Geometry: see drawing. Coordinates: mm, zero at the bounding-box minimum. Round coordinates to 2 decimals unless told otherwise and drop trailing zeros. Loops run counter-clockwise (first coordinate to the right, second up) from the corner with the lowest first, then second, coordinate; pieces in that order, holes last.
(1) Line query: line 1 (X direction, y = 3.75, z = 179) (1 decimal); line 2 (Z direction, x = 157, y = 5) (1 decimal); line 3 (X direction, y = 2.5, z = 171.5) (1 decimal). Output: solid intervals per line, ascending.
(2) First-contact query: pin 1 Ø4 at (x, z) = (17.46, 119.06) entering from +Y; pin 2 Ø6 at (x, z) = (41, 180.5) entering from -Y; pin 3 Ø3 at (y, z) = (2, 55) entering from -X; pin 4 Ø3 at (x, y) = (37, 3) entering from -Z (1 decimal). Flat tips, straight axial feed; report the tip coordinate or a pass-through.
(3) Cut plane C-C, the plane y = 1.25. Output: boundary loops of the cut face in (x, z) (1 decimal), and give its area (3 significant figures).
(4) Cut plane D-D, the plane z = 206. Output: boundary loops of the cut face in (x, y).
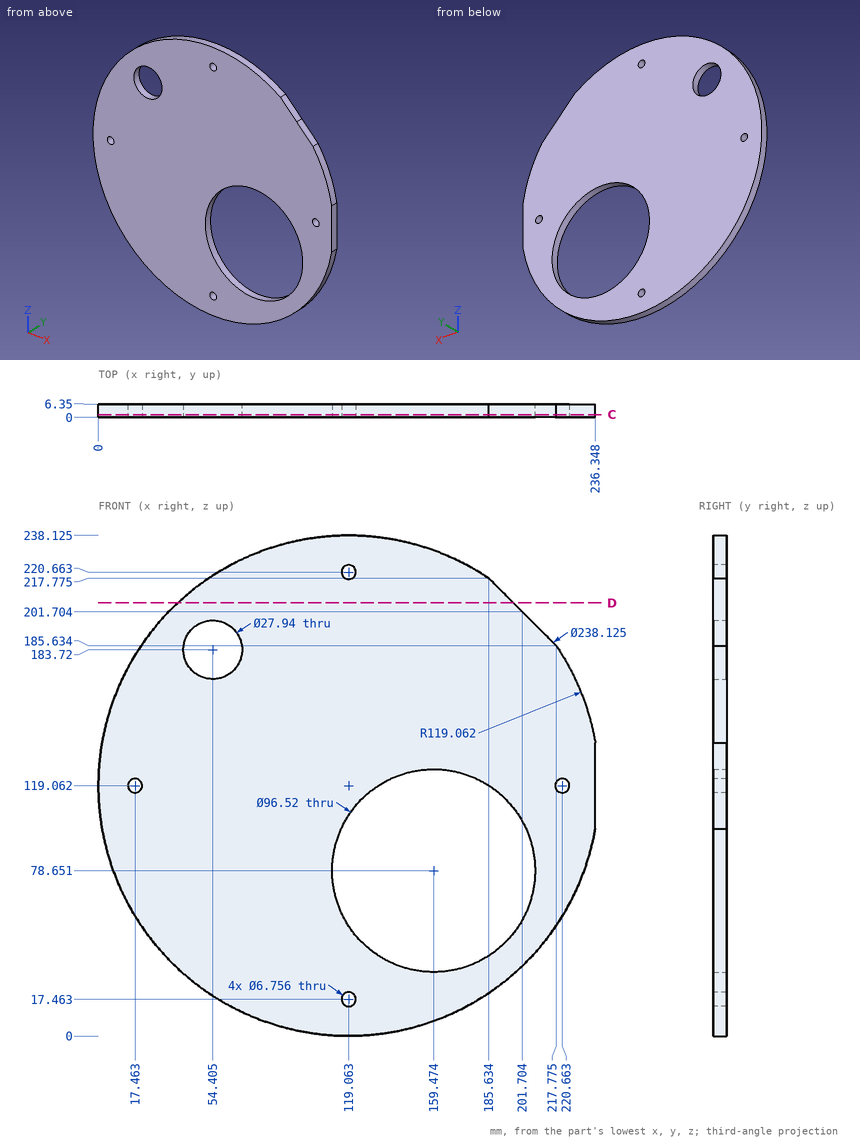
Reported:
1. line 1: x = 16.2 to 41.3, 67.6 to 221.9
1. line 2: z = 6.2 to 30.5, 126.8 to 231.9
1. line 3: x = 12.2 to 47.6, 61.2 to 226
2. pin 1: passes through
2. pin 2: stops at y = 0
2. pin 3: stops at x = 17.76
2. pin 4: stops at z = 31.4
3. outline: (185.6, 217.8) arc R119.1 ccw (long way) to (236.3, 98.6) - (236.3, 139.6) arc R119.1 ccw to (217.8, 185.6) - (201.7, 201.7) - close; hole circle Ø6.8 at (17.5, 119.1); hole circle Ø27.9 at (54.4, 183.7); hole circle Ø96.5 at (159.5, 78.7); hole circle Ø6.8 at (119.1, 17.5); hole circle Ø6.8 at (119.1, 220.7); hole circle Ø6.8 at (220.7, 119.1)
3. area: 36,300 mm2
4. outline: (37.71, 0) - (197.41, 0) - (197.41, 6.35) - (37.71, 6.35) - close
